Autodesk Fusion 360 part; units mm, degrees
sketch "Sketch1" plane through (0, 0, 0) normal (0, 1, 0) x (1, 0, 0)
  line L0 (0, 0) -> (24, 0)
  line L1 (24, 0) -> (24, -4)
  line L2 (24, -4) -> (0, -4)
  line L3 (0, -4) -> (0, 0)
  line L4 (10, 0) -> (14, 0)
  line L5 (14, 0) -> (14, -14)
  line L6 (14, -14) -> (10, -14)
  line L7 (10, -14) -> (10, 0)
  dimension "d1" = 24
  dimension "d2" = 4
  dimension "d3" = 24
  dimension "d4" = 4
  dimension "d5" = 4
  dimension "d6" = 10
  dimension "d7" = 10
extrude "Extrude1" add sketch "Sketch1" along normal blind 4
sketch "Sketch2" plane through (24, 0, 0) normal (1, 0, 0) x (0, 1, 0)
  line L0 (0, 4) -> (0, 0)
  line L1 (0, 0) -> (4, 0)
  line L2 (4, 0) -> (4, 4)
  line L3 (4, 4) -> (0, 4)
  circle A0 centre (2, 2) radius 0.8
  dimension "d10" = 1.6
  dimension "d11" = 2
  dimension "d12" = 2
extrude "Extrude2" cut sketch "Sketch2" against normal blind 24 contours A0
sketch "Sketch3" plane through (0, 0, 14) normal (0, 0, 1) x (-1, 0, 0)
  line L0 (-10, 0) -> (-14, 0)
  line L1 (-14, 0) -> (-14, -4)
  line L2 (-14, -4) -> (-10, -4)
  line L3 (-10, -4) -> (-10, 0)
  circle A0 centre (-12, -2) radius 0.8
  dimension "d15" = 1.6
  dimension "d16" = 2
  dimension "d17" = 2
extrude "Extrude3" cut sketch "Sketch3" against normal blind 10 contours A0
chamfer "Chamfer1" distance 1 angle 45 10 edges at (19, 0, 4) (14, 0, 9) (10, 0, 9) (5, 0, 4) (12, 0, 0) (19, 4, 4) (14, 4, 9) (10, 4, 9) (5, 4, 4) (12, 4, 0)
equation "d1 = 10 mm + 10 mm + 4 mm"
Geometry check sheet. Reference: the model listing, model coordinates, mm. A direction names the side the tool comes from. Round coordinates to 2 decimals unless told otherwise and drop trailing zeros. Write each loop counter-clockwise with the first axis right and the second up, starting at its lowest first coordinate (ties: lowest second). Pieces come first, ordered by that corner, then holes. Notation, with made-up numbers: (12.25, 73) -> (30.25, 73) arc R12 ccw to (30.25, 84) -> close; hole circle Ø9 at (-17, 3.25). An arc over 180 degrees is marked (long way). One line per item, written item: value. Start each with the question number.
(1) Cross-section at C-C, the plane x = 22.75. Record the cut outline in (y, z).
(2) Scan lines: line 1 (Z direction, x = 13.5, y = 2); line 2 (X direction, y = 2, z = 10.5); line 3 (Z direction, x = 2.25, y = 1.6). Record each from-to range of solid material in increasing order. Write a range as [from, to].
(3) Cross-section at B-B, the plane z = 2. Record the cut outline in (x, y), and give its area (3 significant figures).
(4) Go/stop test with flat-tipped pins: pin 1 Ø1.8 at (x, y) = (12, 2) entering from -Z; pin 2 Ø1.6 at (y, z) = (2.5, 7) entering from -X; pin 3 Ø1.6 at (x, y) = (18, 2) entering from +Z; pin 4 Ø1 at (x, z) = (7.5, 5) entering from +Y. Record where each tip stops, or that it passes through.
(5) Cross-section at A-A, the plane y = 2. Record the cut outline in (x, z).
(6) Access from +Z, -Z, +X, -X, +Y, -Y to the whole of each face (thin tool, end or side, straight path). Record for faces 1 (the flat face through (10.5, 0.5, 8.6)), 2 (the flat face through (18.6, 3.5, 3.5)), 3 (the flat face through (10.5, 3.5, 8.6)), 4 (the flat face through (14, 2, 9)), 5 (the flat face through (5, 2, 4)).
(7) Draft check along Y on faces 6 (the flat face through (13.5, 3.5, 8.4)), 7 (the flat face through (12, 2, 0)), 8 (the flat face through (12, 2, 4)). Enter one of: +Y half, -Y half, draft (parallel to the pull), parting line (faces both ways), or undercut.
(8) Cross-section at D-D, the plane z = 12.75. Record the cut outline in (x, y), and give its area (3 significant figures).
Answer:
1. outline: (0, 1) -> (1, 0) -> (3, 0) -> (4, 1) -> (4, 3) -> (3, 4) -> (1, 4) -> (0, 3) -> close; hole circle Ø1.6 at (2, 2)
2. line 1: [0, 1.2], [2.8, 14]
2. line 2: [10, 11.2], [12.8, 14]
2. line 3: [0, 1.31], [2.69, 4]
3. outline: (0, 0) -> (24, 0) -> (24, 1.2) -> (0, 1.2) -> close; (0, 2.8) -> (24, 2.8) -> (24, 4) -> (0, 4) -> close
3. area: 57.6 mm²
4. pin 1: z = 0
4. pin 2: x = 10
4. pin 3: z = 4
4. pin 4: through
5. outline: (0, 0) -> (24, 0) -> (24, 1.2) -> (0, 1.2) -> close; (0, 2.8) -> (24, 2.8) -> (24, 4) -> (14, 4) -> (14, 14) -> (12.8, 14) -> (12.8, 4) -> (11.2, 4) -> (11.2, 14) -> (10, 14) -> (10, 4) -> (0, 4) -> close
6. face 1: +Z, -X, -Y
6. face 2: +Z, +X, +Y
6. face 3: +Z, -X, +Y
6. face 4: +Z, +X, +Y, -Y
6. face 5: +Z, -X, +Y, -Y
7. face 6: +Y half
7. face 7: draft
7. face 8: undercut
8. outline: (10, 1) -> (11, 0) -> (13, 0) -> (14, 1) -> (14, 3) -> (13, 4) -> (11, 4) -> (10, 3) -> close; hole circle Ø1.6 at (12, 2)
8. area: 12.0 mm²
